Geometry: final body of the model. Coordinates: model frame, mm. A direction names the side the tool comes from. Give positions to 0.01 mm unless a question says otherwise; leave off trailing zeros. Loops run counter-clockwise (first coordinate to the right, second up) from the corner with the lowest first, then second, coordinate; pieces in that order, holes last. Notation, with made-up numbers: (8.5, 34) -> (32.5, 34) arc R29 cw to (32.5, 66) -> close; hole circle Ø6 at (-7, 66.5). An arc over 180 degrees is marked (long way). Answer in a Markdown table with one row per item. Add a question column.
1) Section query B-B (y = 2.5). Give the number of separate pieces and of enclosed holes in the cut face, plus the area to 3 significant figures.
2) Section query D-D (z = -27.5). Return the cut outline in (x, y), plus the area to 3 significant figures.
3) Section query A-A (z = -10). Return the cut outline in (x, y).
4) Draft query along X for faces 1 (the cylindrical face through (24.783, 1.479, -14.474)), 2 (the flat face through (-60, 1, -8.936)), 3 (the cylindrical face through (-28.385, 1.479, -27.486)). Return one class per face: +X half, -X half, draft (parallel to the pull), parting line (faces both ways), or undercut.
5) Access query for faces 4 (the flat face through (-16, 3, -15)), 5 (the flat face through (-60, 1, -21.136)). Directions: +Z, -Z, +X, -X, +Y, -Y. A direction counts if a zero-diameter tool reaches every point of the face in a straight line with its end or side. Return the directions, or none.
6) First-contact query: P1, Ø1.5, axis at y = 0.5, z = -12.5, coming from the -X side. Flat tip, straight axial feed; report the tip coordinate or a pass-through.
7) Line query: line 1 (X direction, y = 0.6, z = -17); line 2 (X direction, y = 0.3, z = -19); line 3 (Z direction, x = 2, y = 0.95). Output: solid intervals per line, ascending. Write a range as from..to.
8) Section query C-C (x = -42). Return the cut outline in (y, z), plus the area to 3 significant figures.
```python
from build123d import *

# Parameters (mm, degrees)
SKETCH1_R           = 1.93023
SKETCH1_R_2         = 1.061627907
SKETCH1_R_3         = 0.965116279
SKETCH1_R_4         = 0.96512
SKETCH1_W           = 22.5
SKETCH1_H           = 12.2
BOSS_EXTRUDE1_DEPTH = 3


with BuildPart() as part:
    # Sketch1 → Boss-Extrude1 (new body)
    with BuildSketch(Plane(origin=(0, 0, 0), x_dir=(1, 0, 0), z_dir=(0, 1, 0))):
        with BuildLine():
            ThreePointArc((-66.883539, 26.379856778), (-78.440375529, 14.823020249), (-66.883539, 3.26618372))
            ThreePointArc((-66.883539, 3.26618372), (-28.9420606, 1.724738168), (8.930411, -1.033473673))
            ThreePointArc((8.930411, -1.033473673), (24.786904692, 14.823020019), (8.930411, 30.679513711))
            ThreePointArc((8.930411, 30.679513711), (-28.915651041, 27.455633961), (-66.883539, 26.379856778))
        make_face()
        with Locations((8.930411, 14.823020019)):
            Circle(SKETCH1_R, mode=Mode.SUBTRACT)
        with Locations((-74.238049948, 14.823020249)):
            Circle(SKETCH1_R_2, mode=Mode.SUBTRACT)
        with Locations((-46.438049948, 14.823020249)):
            Circle(SKETCH1_R_2, mode=Mode.SUBTRACT)
        with Locations((2.705411, 14.823020019)):
            Circle(SKETCH1_R_3, mode=Mode.SUBTRACT)
        with Locations((-3.519589, 14.823020019)):
            Circle(SKETCH1_R_3, mode=Mode.SUBTRACT)
        with Locations((15.15541, 14.82302)):
            Circle(SKETCH1_R_4, mode=Mode.SUBTRACT)
        with Locations((21.380409, 14.823020019)):
            Circle(SKETCH1_R_4, mode=Mode.SUBTRACT)
        with Locations((-60.338049948, 15.035810946)):
            Rectangle(SKETCH1_W, SKETCH1_H, mode=Mode.SUBTRACT)
    extrude(amount=BOSS_EXTRUDE1_DEPTH)


solid = part.part
```
Evaluation:
| question | item | result |
|---|---|---|
| 1 | separate pieces | 1 |
| 1 | enclosed holes | 8 |
| 1 | area | 2,290 mm² |
| 2 | outline | (-28.14, 0) -> (18.46, 0) -> (18.46, 3) -> (-28.14, 3) -> close |
| 2 | area | 140 mm² |
| 3 | outline | (-77.39, 0) -> (-71.59, 0) -> (-71.59, 3) -> (-77.39, 3) -> close; (-49.09, 0) -> (24.04, 0) -> (24.04, 3) -> (-49.09, 3) -> close |
| 4 | face 1 | +X half |
| 4 | face 2 | undercut |
| 4 | face 3 | -X half |
| 5 | face 4 | +Z, -Z, +X, -X, +Y |
| 5 | face 5 | +Y, -Y |
| 6 | P1 | x = -78.33 |
| 7 | line 1 | -78.23..-71.59, -49.09..24.64 |
| 7 | line 2 | -77.66..-71.59, -49.09..24.23 |
| 7 | line 3 | -29.93..-15.48, -14.16..0.44 |
| 8 | outline | (0, -26.84) -> (3, -26.84) -> (3, -2.39) -> (0, -2.39) -> close |
| 8 | area | 73.3 mm² |
